```python
from build123d import *

# Parameters (mm, degrees)
SKETCH2_W           = 70
SKETCH2_H           = 12
BOSS_EXTRUDE2_DEPTH = 75
CUT_EXTRUDE2_DEPTH  = 75
FILLET2_R           = 20
SKETCH11_R          = 8
CUT_EXTRUDE9_DEPTH  = 20
SKETCH13_R          = 8
CUT_EXTRUDE10_DEPTH = 107.343782141
CUT_EXTRUDE11_DEPTH = 161.888159912
FILLET3_R           = 12


with BuildPart() as part:
    # Sketch2 → Boss-Extrude2 (new body)
    with BuildSketch(Plane.XY):
        Polygon((12, 48), (0, 48), (0, 0), (64, 0), (64, 48), (52, 48), (52, 20), (12, 20), align=None)
        with Locations((-35, 6)):
            Rectangle(SKETCH2_W, SKETCH2_H)
    extrude(amount=-BOSS_EXTRUDE2_DEPTH)

    # Sketch4 → Cut-Extrude2 (cut)
    with BuildSketch(Plane(origin=(0, 12, 0), x_dir=(1, 0, 0), z_dir=(0, 1, 0))):
        with BuildLine():
            ThreePointArc((-70, 37.5), (-64.142135624, 51.642135624), (-50, 57.5))
            Line((-50, 57.5), (0, 57.5))
            Line((0, 57.5), (0, 75))
            Line((0, 75), (-70, 75))
            Line((-70, 75), (-70, 37.5))
        make_face()
        with BuildLine():
            ThreePointArc((-50, 17.5), (-64.142135624, 23.357864376), (-70, 37.5))
            Line((-70, 37.5), (-70, 0))
            Line((-70, 0), (0, 0))
            Line((0, 0), (0, 17.5))
            Line((0, 17.5), (-50, 17.5))
        make_face()
    extrude(amount=-CUT_EXTRUDE2_DEPTH, mode=Mode.SUBTRACT)

    # Fillet2
    # the kernel refuses this fillet: 20 mm, written as the material it adds along each edge
    with BuildSketch(Plane(origin=(0, 12, -57.5), x_dir=(-1, 0, 0), z_dir=(0, -1, 0))) as fillet2_piece_1:
        with BuildLine():
            CenterArc((19.843134833, 20), FILLET2_R, 187.180755781, 82.819244219)
            Line((0, 17.5), (-0.396862697, 17.45))
            ThreePointArc((-0.396862697, 17.45), (-0.4, 8.75), (-0.4, 0))
            Line((-0.4, 0), (0, -0.4))
            Line((0, -0.4), (19.843134833, -0.4))
            Line((19.843134833, -0.4), (19.843134833, 0))
        make_face()
    extrude(amount=12)
    with BuildSketch(Plane(origin=(0, 12, -17.5), x_dir=(-1, 0, 0), z_dir=(0, -1, 0))) as fillet2_piece_2:
        with BuildLine():
            CenterArc((19.843134833, -20), FILLET2_R, 90, 82.819244219)
            Line((0, -17.5), (-0.396862697, -17.45))
            ThreePointArc((-0.396862697, -17.45), (-0.4, -8.75), (-0.4, 0))
            Line((-0.4, 0), (0, 0.4))
            Line((0, 0.4), (19.843134833, 0.4))
            Line((19.843134833, 0.4), (19.843134833, 0))
        make_face()
    extrude(amount=12)

    # Sketch11 → Cut-Extrude9 (cut)
    with BuildSketch(Plane(origin=(0, 12, 0), x_dir=(1, 0, 0), z_dir=(0, 1, 0))):
        with Locations(Location((-50, 37.5, 0), (0, 0, 180))):
            Circle(SKETCH11_R)
    extrude(amount=-CUT_EXTRUDE9_DEPTH, mode=Mode.SUBTRACT)

    # Sketch13 → Cut-Extrude10 (cut, through all)
    with BuildSketch(Plane(origin=(0, 20, 0), x_dir=(1, 0, 0), z_dir=(0, 1, 0))):
        with Locations(Location((32, 62.5, 0), (0, 0, 180))):
            Circle(SKETCH13_R)
        with Locations(Location((32, 12.5, 0), (0, 0, 180))):
            Circle(SKETCH13_R)
    extrude(amount=-CUT_EXTRUDE10_DEPTH, mode=Mode.SUBTRACT)

    # Sketch14 → Cut-Extrude11 (cut, through all)
    with BuildSketch(Plane(origin=(64, 0, 0), x_dir=(0, 0, -1), z_dir=(1, 0, 0))):
        with BuildLine():
            Line((15.5, 42), (59.5, 42))
            ThreePointArc((59.5, 42), (65.5, 36), (59.5, 30))
            Line((59.5, 30), (15.5, 30))
            ThreePointArc((15.5, 30), (9.5, 36), (15.5, 42))
        make_face()
    extrude(amount=-CUT_EXTRUDE11_DEPTH, mode=Mode.SUBTRACT)

    # Fillet3
    fillet3_edges = [part.edges().sort_by_distance(p)[0] for p in [
        (58, 48, 0),
        (6, 48, 0),
        (6, 48, -75),
        (58, 48, -75),
    ]]
    fillet(fillet3_edges, radius=FILLET3_R)


solid = part.part
```
Geometry check sheet. Reference: the model listing, model coordinates, mm. A direction names the side the tool comes from. Coordinates: 2 decimals unless noted, no trailing zeros. Write each loop counter-clockwise with the first axis right and the second up, starting at its lowest first coordinate (ties: lowest second). Pieces come first, ordered by that corner, then holes. Notation, with made-up numbers: M 6,85.5 L 62,85.5 A26 cw 62,105.5 Z; hole C 84,25 d3. An arc over 180 degrees is marked long. One line per item, written item: value. Start each with the question number.
(1) Depth check by flat-ended pin: pin 1 (9.5 mm diameter, centred on x = -42.5, y = 5.5, fed in from +Z); pin 2 (10 mm diameter, centred on x = 38, z = -10.5, fed in from +Y); pin 3 (14.5 mm diameter, centred on x = 32, z = -62.5, fed in from -Y); pin 4 (6 mm diameter, centred on x = -11, z = -44, fed in from +Y). Enter the tip coordinate at first touch or a pass-through.
(2) Scan lines: line 1 along Z through (x, y) = (32, 10.25); line 2 along Y through (x, z) = (1, -30); line 3 along X through (y, z) = (8, -37). Record each from-to range of solid material in increasing order. Write a range as [from, to].
(3) Sectioned sample at C-C, the plane z = -68. Enter the section's corners in (x, y), and give its area (3 significant figures).
(4) Release check for a two-part mould opening along X. For faces 6 (the face through (38.349, 10.14, -17.368)), 7 (the face through (58, 42, -37)), 8 (the face through (-6.5, 6.1, -62.6)) record: released by +X, released by -X, zero draft, split by the parting line, or undercut.
(5) Sectioned sample at B-B, the plane x = 32. Enter the section's corners in (y, z).
(6) Sectioned sample at A-A, the plane y = 24.5. Enter the section's corners in (x, z), and give its area (3 significant figures).
(7) Tool access check on faces 1 (the face through (-35, 6, -57.5)), 2 (the face through (32, 20, -37)), 3 (the face through (-35, 12, -38)), 4 (the face through (33.041, 10.14, -54.568)), 5 (the face through (6, 30, -38)). Record the directions out of +Z, -Z, +X, -X, +Y, -Y that give a thin tool (end or side, any length) a straight path to the whole face; none if there is none.
(8) Sectioned sample at D-D, the plane x = -48. Enter the section's corners in (y, z), and give its area (3 significant figures).
Filled sheet:
1. pin 1: z = -17.5
1. pin 2: y = 20
1. pin 3: through
1. pin 4: y = 12
2. line 1: [-75, -70.5], [-54.5, -20.5], [-4.5, 0]
2. line 2: [0, 30], [42, 48]
2. line 3: [-69.99, -57.98], [-42.02, 64]
3. outline: M -2.24,0 L 26.19,0 L 26.19,20 L 12,20 L 12,46.91 L 0,46.91 L 0,12 L -2.24,12 Z; M 37.81,0 L 64,0 L 64,46.91 L 52,46.91 L 52,20 L 37.81,20 Z
3. area: 1,720 mm²
4. face 6: undercut
4. face 7: zero draft
4. face 8: released by -X
5. outline: M 0,-75 L 20,-75 L 20,-70.5 L 0,-70.5 Z; M 0,-54.5 L 20,-54.5 L 20,-20.5 L 0,-20.5 Z; M 0,-4.5 L 20,-4.5 L 20,0 L 0,0 Z
6. outline: M 0,-75 L 12,-75 L 12,0 L 0,0 Z; M 52,-75 L 64,-75 L 64,0 L 52,0 Z
6. area: 1,800 mm²
7. face 1: -Z, -X, +Y, -Y
7. face 2: +Z, -Z, +Y
7. face 3: +Z, -Z, -X, +Y
7. face 4: +Y, -Y
7. face 5: +X, -X
8. outline: M 0,-57.5 L 12,-57.5 L 12,-45.25 L 0,-45.25 Z; M 0,-29.75 L 12,-29.75 L 12,-17.5 L 0,-17.5 Z
8. area: 294 mm²
